Here's how the part is built. I have some questions about the finished solid (model axes, mm). A direction names the side the tool comes from. Coordinates: 2 decimals unless noted, no trailing zeros. Write each loop counter-clockwise with the first axis right and the second up, starting at its lowest first coordinate (ties: lowest second). Pieces come first, ordered by that corner, then holes. Notation, with made-up numbers: (66, 30.25) -> (83, 30.25) arc R21 ccw to (83, 64.25) -> close; hole circle Ø10 at (-9, -5.75). An arc over 180 degrees is marked (long way). Use a Markdown table: item, result. Add a question column.
```python
from build123d import *

# Parameters (mm, degrees)
F0_W     = 90
F0_H     = 10
F0_W_2   = 10
F0_H_2   = 26
F1_DEPTH = 5
F2_DEPTH = 5
F3_DEPTH = 57.5


with BuildPart() as f1:
    # F0 (on Top) → F1 (new body)
    with BuildSketch(Plane.XY):
        with Locations((0, 18)):
            Rectangle(F0_W, F0_H)
        with Locations((-50, 0)):
            Rectangle(F0_W_2, F0_H_2)
        with Locations((-50, 18)):
            Rectangle(F0_W_2, F0_H)
        with Locations((50, 0)):
            Rectangle(F0_W_2, F0_H_2)
        with Locations((50, 18)):
            Rectangle(F0_W_2, F0_H)
        with Locations((-50, -18)):
            Rectangle(F0_W_2, F0_H)
        with Locations((0, -18)):
            Rectangle(F0_W, F0_H)
        with Locations((50, -18)):
            Rectangle(F0_W_2, F0_H)
    extrude(amount=-F1_DEPTH)

    # F0 (on Top) → F2 (join)
    with BuildSketch(Plane.XY):
        Rectangle(F0_W, F0_H_2)
    extrude(amount=-F2_DEPTH)

    # F0 (on Top) → F3 (join)
    with BuildSketch(Plane.XY):
        with Locations((-50, 18)):
            Rectangle(F0_W_2, F0_H)
        with Locations((50, 18)):
            Rectangle(F0_W_2, F0_H)
        with Locations((50, -18)):
            Rectangle(F0_W_2, F0_H)
        with Locations((-50, -18)):
            Rectangle(F0_W_2, F0_H)
    extrude(amount=-F3_DEPTH)


solid = f1.part
```
Q1. Which directions (+Z, -Z, +X, -X, +Y, -Y) give clear straight access to the entire face, cutting with the end or side of a thin tool? Please do faces 1 (the flat face through (-50, -18, -57.5)), 2 (the flat face through (45, -18, -31)), 3 (the flat face through (50, 13, -31)).
Q2. Suppose I cut it at D-D, the plane y = -4. Write out the boundary of the cut face in (x, z).
Q3. Suppose I cut it at C-C, the plane x = -39.5. Write out the boundary of the cut face in (y, z).
Q4. Thinking about a two-plate mould opening in X: for faces 4 (the flat face through (55, -16, -28)), 5 (the flat face through (-45, -18, -31)), 6 (the flat face through (50, 18, -57.5)), which applies, released by +X, released by -X, zero draft, split by the parting line, or undercut?
Q5. Please list where these lines run through material, in increasing order: line 1 (X direction, y = 18, z = -50); line 2 (Z direction, x = 34, y = 12.5); line 3 (Y direction, x = 46, z = -8).
Q6. Will this pin go through, and if not, where does the flat tip stop? pin 1 (3 mm diameter, centred on y = -10, z = -29, fed in from +X).
Q7. Suppose I cut it at A-A, the plane z = -38. Write out the boundary of the cut face in (x, y).
Q8. Suppose I cut it at B-B, the plane y = 16.5. Write out the boundary of the cut face in (x, z).
Answer key:
| question | item | result |
|---|---|---|
| 1 | face 1 | -Z, +X, -X, +Y, -Y |
| 1 | face 2 | -Z, +Y, -Y |
| 1 | face 3 | -Z, +X, -X |
| 2 | outline | (-55, -5) -> (55, -5) -> (55, 0) -> (-55, 0) -> close |
| 3 | outline | (-23, -5) -> (23, -5) -> (23, 0) -> (-23, 0) -> close |
| 4 | face 4 | released by +X |
| 4 | face 5 | undercut |
| 4 | face 6 | zero draft |
| 5 | line 1 | x = -55 to -45, 45 to 55 |
| 5 | line 2 | z = -5 to 0 |
| 5 | line 3 | y = -23 to -13, 13 to 23 |
| 6 | pin 1 | passes through |
| 7 | outline | (-55, -23) -> (-45, -23) -> (-45, -13) -> (-55, -13) -> close; (-55, 13) -> (-45, 13) -> (-45, 23) -> (-55, 23) -> close; (45, -23) -> (55, -23) -> (55, -13) -> (45, -13) -> close; (45, 13) -> (55, 13) -> (55, 23) -> (45, 23) -> close |
| 8 | outline | (-55, -57.5) -> (-45, -57.5) -> (-45, -5) -> (45, -5) -> (45, -57.5) -> (55, -57.5) -> (55, 0) -> (-55, 0) -> close |
